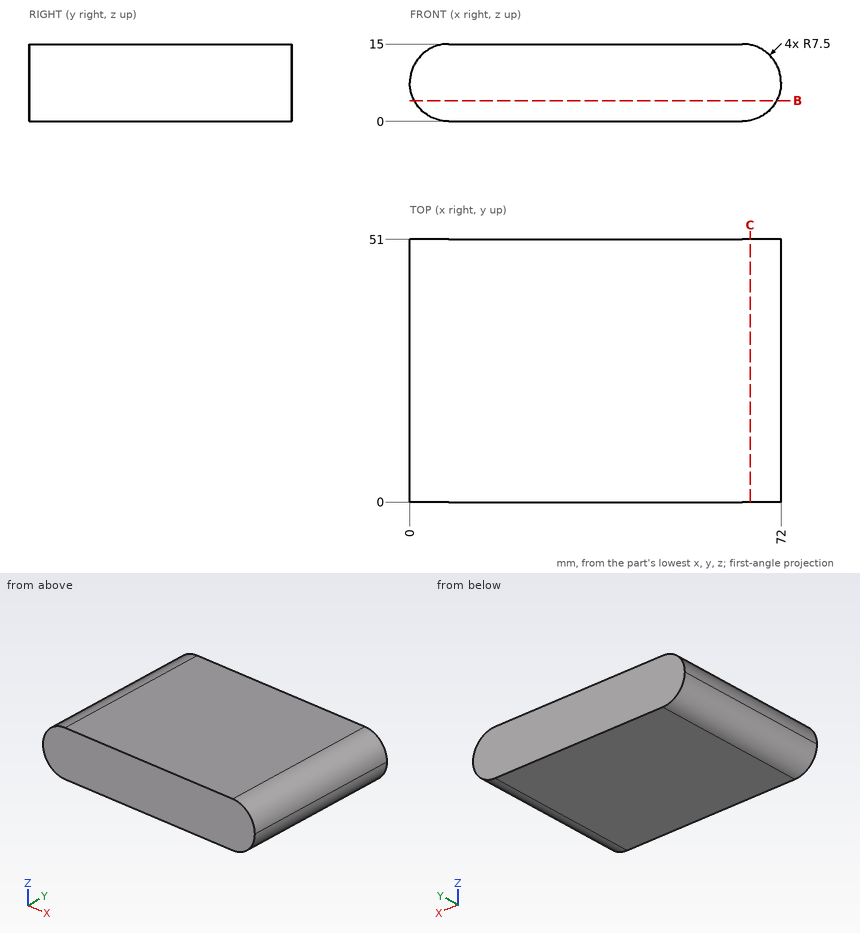
Geometry check sheet. Reference: drawing and pictorial views, mm from the part's lowest x, y, z. Round coordinates to 2 decimals unless told otherwise and drop trailing zeros. Loops run counter-clockwise (first coordinate to the right, second up) from the corner with the lowest first, then second, coordinate; pieces in that order, holes last. Notation, with made-up numbers: M 20.25,39.25 L 68.25,39.25 A22 ccw 68.25,73.25 Z; hole C 10,14.25 d7. An arc over 180 degrees is marked long. One line per item, written item: value.
(1) Sectioned sample at B-B, the plane z = 4. Record the cut outline in (x, y), then the cut area to 3 significant figures.
Computed values:
outline: M 0.87,0 L 71.13,0 L 71.13,51 L 0.87,51 Z
area: 3,580 mm^2
(2) Thickness scan on line 1 (X direction, y = 4, z = 8.5); line 2 (X direction, y = 32, z = 12); line 3 (Z direction, x = 4, y = 18). Record the ranges inside material, lowest first.
Computed values:
line 1: x = 0.07 to 71.93
line 2: x = 1.5 to 70.5
line 3: z = 0.87 to 14.13
(3) Sectioned sample at C-C, the plane x = 66. Record the cut outline in (y, z).
Computed values:
outline: M 0,0.15 L 51,0.15 L 51,14.85 L 0,14.85 Z
(4) Depth check by flat-ended pin: pin 1 Ø8 at (y, z) = (28, 12) entering from -X; pin 2 Ø1 at (y, z) = (10.5, 11.5) entering from -X; pin 3 Ø2 at (y, z) = (34.5, 5.5) entering from +X. Enter the tip coordinate at first touch or a pass-through.
Computed values:
pin 1: stops at x = 0.02
pin 2: stops at x = 0.87
pin 3: stops at x = 71.93
